Geometry: final body of the model. Coordinates: model frame, mm. Face numbers are marked on the shaded views. A direction names the side the tool comes from. Give positions to 0.01 mm unless a question says otherwise; leave off trailing zeros. Order: outer loops, then holes, each group sorted by start corner. A loop starts at its lowest first (then second) coordinate and runs counter-clockwise, first axis right, second up. Notation, with made-up numbers: M -5,-34.5 L 13,-34.5 A20 ccw 13,-14.5 Z; hole C 22,-25.75 d6. An arc over 180 degrees is marked long. Use CSV: the item, a comma, the result in double quotes.
```python
from build123d import *

# Parameters (mm, degrees)
SKETCH1_W                = 20.576303651
SKETCH1_H                = 2.09043177
BOSS_EXTRUDE1_DEPTH      = 30
BOSS_EXTRUDE1_DEPTH_BACK = 20
SKETCH2_W                = 20.576303651
SKETCH2_H                = 18.581877963
BOSS_EXTRUDE2_DEPTH      = 3
SKETCH3_W                = 20.576303651
SKETCH3_H                = 3
BOSS_EXTRUDE3_DEPTH      = 20
SKETCH4_W                = 20.576303651
SKETCH4_H                = 2.723460459
BOSS_EXTRUDE4_DEPTH      = 27


with BuildPart() as part:
    # Sketch1 → Boss-Extrude1 (new body, two sides)
    with BuildSketch(Plane.XY.offset(195.567247699)) as boss_extrude1_sk:
        with Locations((100.659362947, 26.580882383)):
            Rectangle(SKETCH1_W, SKETCH1_H)
    extrude(amount=BOSS_EXTRUDE1_DEPTH)
    extrude(boss_extrude1_sk.sketch, amount=-BOSS_EXTRUDE1_DEPTH_BACK)

    # Sketch2 → Boss-Extrude2 (add)
    with BuildSketch(Plane.XY.offset(195.567247699)):
        with Locations((100.659362947, 36.91703725)):
            Rectangle(SKETCH2_W, SKETCH2_H)
    extrude(amount=BOSS_EXTRUDE2_DEPTH)

    # Sketch3 → Boss-Extrude3 (add)
    with BuildSketch(Plane.XZ.offset(-25.535666498)):
        with Locations((100.659362947, 197.067247699)):
            Rectangle(SKETCH3_W, SKETCH3_H)
    extrude(amount=BOSS_EXTRUDE3_DEPTH)

    # Sketch4 → Boss-Extrude4 (add)
    with BuildSketch(Plane.XY.offset(198.567247699)):
        with Locations((100.659362947, 6.897396728)):
            Rectangle(SKETCH4_W, SKETCH4_H)
    extrude(amount=BOSS_EXTRUDE4_DEPTH)


solid = part.part
```
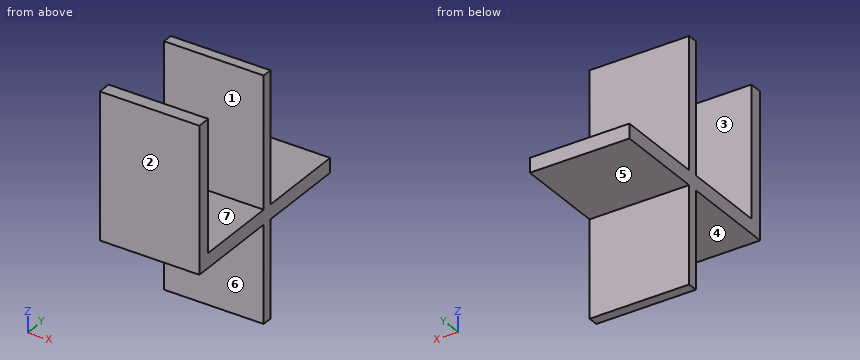
1. Section C-C, the plane y = 38.5. Return the cut outline in (x, z).
Answer:
outline,"M 90.37,195.57 L 110.95,195.57 L 110.95,198.57 L 90.37,198.57 Z"
2. Line query: line 1 (Y direction, x = 92, z = 223); line 2 (Z direction, x = 104.25, y = 16); line 3 (Y direction, x = 104.5, z = 195). Output: solid intervals per line, ascending.
Answer:
line 1,"5.54 to 8.26, 25.54 to 27.63"
line 2,"195.57 to 198.57"
line 3,"25.54 to 27.63"
3. Pull-direction query (Y, two-part tool) for the marked faces 1, 2, 3 and 4; classes: +Y half, -Y half, draft (parallel to the pull), parting line (faces both ways), or undercut.
Answer:
face 1,"undercut"
face 2,"-Y half"
face 3,"undercut"
face 4,"draft"
4. Section A-A, the plane z = 205.5. Return the cut outline in (x, y).
Answer:
outline,"M 90.37,5.54 L 110.95,5.54 L 110.95,8.26 L 90.37,8.26 Z; M 90.37,25.54 L 110.95,25.54 L 110.95,27.63 L 90.37,27.63 Z"
5. Section B-B, the plane x = 101. Return the cut outline in (y, z).
Answer:
outline,"M 5.54,195.57 L 25.54,195.57 L 25.54,175.57 L 27.63,175.57 L 27.63,195.57 L 46.21,195.57 L 46.21,198.57 L 27.63,198.57 L 27.63,225.57 L 25.54,225.57 L 25.54,198.57 L 8.26,198.57 L 8.26,225.57 L 5.54,225.57 Z"
6. Reachability of the marked faces 5, 6 and 7 from +Z, -Z, +X, -X, +Y, -Y: full face, straight path, thin tool, end or side. Return the list, or none.
Answer:
face 5,"-Z, +X, -X, +Y"
face 6,"-Z, +X, -X, -Y"
face 7,"+Z, +X, -X"
7. Section D-D, the plane z = 186.5. Return the cut outline in (x, y).
Answer:
outline,"M 90.37,25.54 L 110.95,25.54 L 110.95,27.63 L 90.37,27.63 Z"
8. Pin query (flat end, axial travel): pin 1 Ø6 at (x, y) = (99.5, 16) entering from -Z; pin 2 Ø10 at (x, z) = (104.5, 181) entering from +Y; pin 3 Ø3 at (y, z) = (11.5, 214) entering from -X; pin 4 Ø9.5 at (x, y) = (97.5, 37) entering from +Z. Return the tip coordinate at first contact, or that it passes through.
Answer:
pin 1,"z = 195.57"
pin 2,"y = 27.63"
pin 3,"through"
pin 4,"z = 198.57"
